```python
from build123d import *

# Parameters (mm, degrees)
F0_R     = 13
F0_R_2   = 5
F1_DEPTH = 4
F2_R     = 11
F2_R_2   = 6.5
F4_DEPTH = 1
F3_R     = 11
F3_R_2   = 6.5
F5_DEPTH = 1
F6_SIZE  = 0.5


with BuildPart() as f1:
    # F0 (on Front) → F1 (new body, symmetric)
    with BuildSketch(Plane.XZ):
        Circle(F0_R)
        Circle(F0_R_2, mode=Mode.SUBTRACT)
    extrude(amount=F1_DEPTH, both=True)

    # F2 (on face) → F4 (cut)
    with BuildSketch(Plane(origin=(0, 4, 0), x_dir=(-1, 0, 0), z_dir=(0, 1, 0))):
        Circle(F2_R)
        Circle(F2_R_2, mode=Mode.SUBTRACT)
    extrude(amount=-F4_DEPTH, mode=Mode.SUBTRACT)

    # F3 (on face) → F5 (cut)
    with BuildSketch(Plane.XZ.offset(4)):
        Circle(F3_R)
        Circle(F3_R_2, mode=Mode.SUBTRACT)
    extrude(amount=-F5_DEPTH, mode=Mode.SUBTRACT)

    # F6
    f6_edges = [f1.edges().sort_by_distance(p)[0] for p in [
        (-13, 4, 0),
        (-13, -4, 0),
        (-5, -4, 0),
        (-5, 4, 0),
        (6.5, 4, 0),
        (11, 4, 0),
        (-11, -4, 0),
        (-6.5, -4, 0),
    ]]
    chamfer(f6_edges, length=F6_SIZE)


solid = f1.part
```
The listing builds one solid part. Answer for the finished solid, in the listing's coordinates (mm). A direction names the side the tool comes from. Give positions to 0.01 mm unless a question says otherwise; leave off trailing zeros. Loops run counter-clockwise (first coordinate to the right, second up) from the corner with the lowest first, then second, coordinate; pieces in that order, holes last. Notation, with made-up numbers: M -36.5,-29.75 L 11.5,-29.75 A12 ccw 11.5,-23.75 Z; hole C -28.5,86.5 d8. An arc over 180 degrees is marked long. One line per item, written item: value.
1. For faces 1 (the face through (2.38, 3.25, -10.74)), 2 (the face through (11, -4, -4)), 3 (the face through (-2.38, -3.25, -10.74)), determine the directions among +Z, -Z, +X, -X, +Y, -Y from which every point of the face is accessible in a straight line to the end or side of a thin tool.
Found:
face 1: +Y
face 2: +Z, -Z, +X, -X, -Y
face 3: -Y
2. For a pull along Z with two mould halves and no side action, classify faces 4 (the face through (-5, 3, -5)), 5 (the face through (-1.08, 0.05, -4.88)), 6 (the face through (11, 4, -4)) as pulls with the +Z half, pulls with the -Z half, needs draft (parallel to the pull), parting line crosses it, or undercut.
Found:
face 4: undercut
face 5: undercut
face 6: needs draft
3. Find the intervals of material crossed by probe 1 along Z at (x, y) = (0, 3.25); probe 2 along Y at (x, z) = (-6.25, 9); probe 3 along X at (y, z) = (2.75, -1.25), in increasing order.
Found:
probe 1: -13 to -11, -6.5 to -5, 5 to 6.5, 11 to 13
probe 2: -3 to 3
probe 3: -12.94 to -4.84, 4.84 to 12.94
4. Section A-A on y = -1.25 is taken. Determine the outline of the cut face in (x, z), plus the area to 3 significant figures.
Found:
outline: C 0,0 d26; hole C 0,0 d10
area: 452 mm^2
